Read the model definition and answer for the solid it produces. Units are mm, in the model's axes. Face numbers are marked on the shaded views. A direction names the side the tool comes from. Give positions to 0.01 mm unless a question says otherwise; leave off trailing zeros. Order: outer loops, then holes, each group sorted by start corner. A loop starts at its lowest first (then second) coordinate and runs counter-clockwise, first axis right, second up. Notation, with made-up numbers: (-2, 85) - (31, 85) arc R22 cw to (31, 124) - close; hole circle Ø4 at (58, 17.25). An arc over 180 degrees is marked (long way). Use a Markdown table: item, result. Add a question column.
1. Which of the six approach directions +Z, -Z, +X, -X, +Y, -Y give full straight-line access (tool end or side, diameter ignored) to the marked faces 1 and 2?
2. For a pull along X with two mould halves and no side action, classify the marked faces 3, 4 and 5 as released by +X, released by -X, zero draft, split by the parting line, or undercut.
3. Consider L1, parallel to X at y = 1, z = 2; L2, parallel to Z at x = 0, y = 12.35; L3, parallel to Z at x = 10.5, y = 2.75. Determine where each line is inside the solid, lowest interval first.
4. Flat-ended cylindrical pins translate along their axes: P1, Ø1, axis at y = 5, z = 7, coming from the +X side; P2, Ø7.5, axis at x = -12, z = 7.5, coming from the +Y side; P3, Ø1.5, axis at y = 8, z = 6, coming from the +X side. Find the tip coordinate at first contact, or state that the pin passes through.
5. A cutting plane is placed at A-A on x = 0. Determine the outline of the cut face in (y, z), and give its area (3 significant figures).
6. A cutting plane is placed at B-B on z = 7. State how many separate pieces and enclosed holes the cut face has, and give its area (3 significant figures).
7. A cutting plane is placed at D-D on z = 9.5. Determine the outline of the cut face in (x, y), and give its area (3 significant figures).
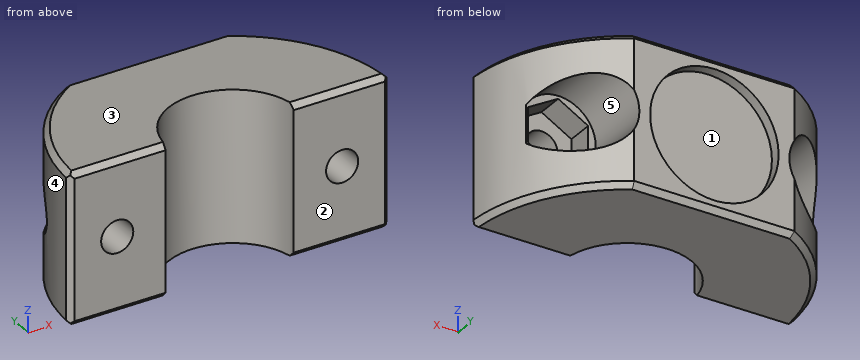
Autodesk Fusion 360 part; units mm, degrees
sketch "スケッチ2" plane through (0, 0, 0) normal (0, 0, 1) x (1, 0, 0)
  line L0 (0, 0.5) -> (0, -0.5)
  arc A0 (-7.4833, 13) -> (-14.9917, 0.4998) centre (0, 0) ccw
  line L1 (-14.9917, 0.4998) -> (-5.9791, 0.4998)
  line L2 (5.9791, 0.4998) -> (14.9917, 0.4998)
  arc A1 (5.9791, 0.4998) -> (-5.9791, 0.4998) centre (0, 0) ccw
  arc A2 (14.9917, 0.4998) -> (7.4833, 13) centre (0, 0) ccw
  line L3 (0, 13) -> (7.4833, 13)
  line L4 (-7.4833, 13) -> (0, 13)
extrude "押し出し1" add sketch "スケッチ2" along normal blind 14
sketch "スケッチ4" plane through (0, 13, 0) normal (0, 1, 0) x (-1, 0, 0)
  line L0 (-7.4833, 0) -> (7.4833, 0)
  line L1 (7.4833, 0) -> (7.4833, 14)
  line L2 (7.4833, 14) -> (-7.4833, 14)
  line L3 (-7.4833, 14) -> (-7.4833, 0)
  circle A0 centre (0, 7) radius 6
  dimension "d7" = 12
extrude "押し出し2" cut sketch "スケッチ4" against normal blind 1 contours A0
sketch "スケッチ5" plane through (0, 0, 0) normal (0, 1, 0) x (1, 0, 0)
  line L0 (0, 1) -> (0, -15)
  line L1 (15, -7) -> (10.5, -7)
  circle A0 centre (10.5, -7) radius 1.5
  circle A1 centre (-10.5, -7) radius 1.5
  dimension "d10" = 4.5
extrude "押し出し3" cut sketch "スケッチ5" along normal blind 13
sketch "スケッチ6" plane through (0, 13, 0) normal (0, 1, 0) x (-1, 0, 0)
  circle A0 centre (0, 7) radius 6
  line L0 (-7.4833, 0) -> (7.4833, 0)
  line L1 (7.4833, 0) -> (7.4833, 14)
  line L2 (7.4833, 14) -> (-7.4833, 14)
  line L3 (-7.4833, 14) -> (-7.4833, 0)
  circle A1 centre (10.5, 7) radius 3.5
  line L4 (-7.7, 8.6166) -> (-10.5, 10.2332)
  line L5 (-10.5, 10.2332) -> (-13.3, 8.6166)
  line L6 (-13.3, 8.6166) -> (-13.3, 5.3834)
  line L7 (-13.3, 5.3834) -> (-10.5, 3.7668)
  line L8 (-10.5, 3.7668) -> (-7.7, 5.3834)
  line L9 (-7.7, 5.3834) -> (-7.7, 8.6166)
  point P0 (10.5, 7)
  point P1 (-10.5, 7)
  point P2 (-10.5, 7)
extrude "押し出し4" cut sketch "スケッチ6" against normal blind 9 contours L1 A1 | L1 A1 | L4 L5 L6 L7 L8 L9
sketch "スケッチ7" plane through (13.3, 0, 0) normal (-1, 0, 0) x (0, -1, 0)
  line L0 (-6.9361, 8.6166) -> (-6.9361, 5.3834)
  line L1 (-6.9361, 5.3834) -> (-4, 5.3834)
  line L2 (-4, 5.3834) -> (-4, 8.6166)
  line L3 (-4, 8.6166) -> (-6.9361, 8.6166)
chamfer "面取り1" distance 0.5 angle 45 8 edges at (0, 13, 0) (-12.8586, 7.7237, 0) (-14.9917, 0.4998, 7) (-12.8586, 7.7237, 14) (0, 13, 14) (12.8586, 7.7237, 14) (12.8586, 7.7237, 0) (14.9917, 0.4998, 7)
sketch "スケッチ8" plane through (0, 13, 0) normal (0, 1, 0) x (-1, 0, 0)
  circle A0 centre (0, 7) radius 6
  line L0 (7.4833, 13.5) -> (-7.4833, 13.5)
  line L1 (-7.4833, 13.5) -> (-7.4833, 0.5)
  line L2 (-7.4833, 0.5) -> (7.4833, 0.5)
  line L3 (7.4833, 0.5) -> (7.4833, 5.2253)
  arc A1 (7.4833, 8.7747) -> (7.4833, 5.2253) centre (10.5, 7) ccw
  line L4 (7.4833, 8.7747) -> (7.4833, 13.5)
  circle A2 centre (-10.5, 7) radius 3.5
  point P0 (-10.5, 7)
  dimension "d18" = 7
extrude "押し出し5" cut sketch "スケッチ8" against normal blind 6.5 contours L1 A2 | L1 A2
chamfer "面取り2" distance 0.5 angle 45 4 edges at (-10.2353, 0.4998, 14) (-10.2353, 0.4998, 0) (10.2353, 0.4998, 0) (10.2353, 0.4998, 14)
sketch "スケッチ9" plane through (0, 0, 0) normal (0, 1, 0) x (1, 0, 0)
  line L0 (20, -7) -> (-20, -7)
Output values:
| question | item | result |
|---|---|---|
| 1 | face 1 | +Y |
| 1 | face 2 | +Z, -Z, +X, -X, -Y |
| 2 | face 3 | zero draft |
| 2 | face 4 | released by -X |
| 2 | face 5 | undercut |
| 3 | L1 | -14.97 to -5.92, 5.92 to 14.97 |
| 3 | L2 | 0 to 1, 13 to 14 |
| 3 | L3 | 0 to 5.5, 8.5 to 14 |
| 4 | P1 | x = 14.31 |
| 4 | P2 | y = 11.52 |
| 4 | P3 | x = 7.47 |
| 5 | outline | (6, 0) - (12.5, 0) - (13, 0.5) - (13, 1) - (12, 1) - (12, 13) - (13, 13) - (13, 13.5) - (12.5, 14) - (6, 14) - close |
| 5 | area | 85.8 mm² |
| 6 | separate pieces | 3 |
| 6 | enclosed holes | 0 |
| 6 | area | 150 mm² |
| 7 | outline | (-14.97, 1) - (-14.49, 0.5) - (-5.98, 0.5) arc R6 cw to (5.98, 0.5) - (14.49, 0.5) - (14.97, 1) arc R15 ccw to (12.95, 7.57) - (12.95, 6.5) - (11.77, 6.5) - (11.77, 4) - (9.23, 4) - (9.23, 6.5) - (8.05, 6.5) - (8.05, 12.66) arc R15 ccw to (7.48, 13) - (5.45, 13) - (5.45, 12) - (-5.45, 12) - (-5.45, 13) - (-7.48, 13) arc R15 ccw to (-8.05, 12.66) - (-8.05, 4) - (-12.95, 4) - (-12.95, 7.57) arc R15 ccw to start |
| 7 | area | 199 mm² |
